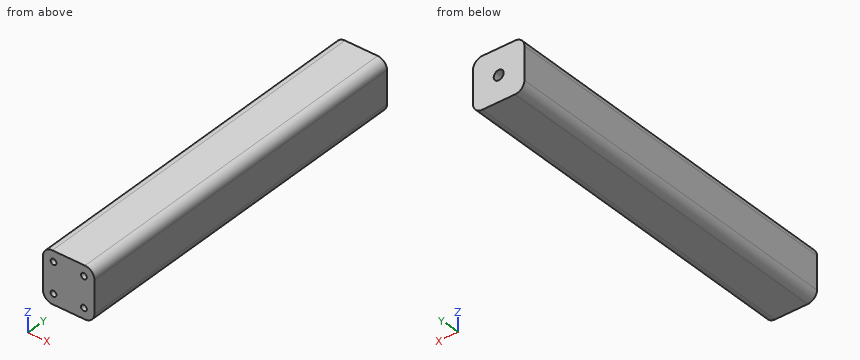
from build123d import *

# Parameters (mm, degrees)
SKETCH_2_W              = 44
SKETCH_2_H              = 44
EXTRUDE_1_DEPTH         = 310
HOLE_WIZARD_M10_1_D     = 8.5
HOLE_WIZARD_M10_1_DEPTH = 25
HOLE_WIZARD_M10_1_TIP   = 2.553657631
HOLE_WIZARD_M6_1_D      = 5
HOLE_WIZARD_M6_1_DEPTH  = 40
HOLE_WIZARD_M6_1_TIP    = 1.502151548
FILLET_1_R              = 8


with BuildPart() as part:
    # 草图2 → 凸台-拉伸1 (new body)
    with BuildSketch(Plane(origin=(0, 0, 0), x_dir=(1, 0, 0), z_dir=(0, 1, 0))):
        with Locations((-0.001355374, -3.30438103)):
            Rectangle(SKETCH_2_W, SKETCH_2_H)
    extrude(amount=EXTRUDE_1_DEPTH)

    # M10 螺纹孔1
    with Locations(Plane(origin=(0, 310, 0), x_dir=(1, 0, 0), z_dir=(0, 1, 0))):
        with Locations((-0.001355374, -3.30438103)):
            Hole(HOLE_WIZARD_M10_1_D / 2, depth=HOLE_WIZARD_M10_1_DEPTH)
            with Locations((0, 0, -(HOLE_WIZARD_M10_1_DEPTH + HOLE_WIZARD_M10_1_TIP / 2))):  # 118° drill point
                Cone(0, HOLE_WIZARD_M10_1_D / 2, HOLE_WIZARD_M10_1_TIP, mode=Mode.SUBTRACT)

    # M6 螺纹孔1
    with Locations(Plane(origin=(-13.001355374, 0, 16.30438103), x_dir=(0, 0, -1), z_dir=(0, -1, 0))):
        with Locations((0, 0), (0, 26), (26, 26), (26, 0)):
            Hole(HOLE_WIZARD_M6_1_D / 2, depth=HOLE_WIZARD_M6_1_DEPTH)
            with Locations((0, 0, -(HOLE_WIZARD_M6_1_DEPTH + HOLE_WIZARD_M6_1_TIP / 2))):  # 118° drill point
                Cone(0, HOLE_WIZARD_M6_1_D / 2, HOLE_WIZARD_M6_1_TIP, mode=Mode.SUBTRACT)

    # 圆角1
    fillet_1_edges = [part.edges().sort_by_distance(p)[0] for p in [
        (-22.001355374, 155, -18.69561897),
        (21.998644626, 155, -18.69561897),
        (21.998644626, 155, 25.30438103),
        (-22.001355374, 155, 25.30438103),
    ]]
    fillet(fillet_1_edges, radius=FILLET_1_R)


solid = part.part
The listing builds one solid part. Answer for the finished solid, in the listing's coordinates (mm). Coordinates: 2 decimals unless noted, no trailing zeros. Write each loop counter-clockwise with the first axis right and the second up, starting at its lowest first coordinate (ties: lowest second). Pieces come first, ordered by that corner, then holes. Notation, with made-up numbers: M 39.25,-17.5 L 86.25,-17.5 A31 ccw 86.25,19.5 Z; hole C -19.75,14.5 d1. An arc over 180 degrees is marked long. Use one line per item in the form item = value.
Item 1: Find the intervals of material crossed by probe 1 along Z at (x, y) = (-12.5, 18); probe 2 along X at (y, z) = (31.5, 16); probe 3 along X at (y, z) = (20, -8.5), in increasing order.
Model answer:
probe_1 = -18.7 to -12.14, -7.25 to 13.86, 18.75 to 25.3
probe_2 = -22 to -15.48, -10.52 to 10.52, 15.48 to 22
probe_3 = -22 to -15.2, -10.81 to 10.8, 15.19 to 22
Item 2: Given P1, Ø4, axis at x = 13, z = -9.7, coming from the -Y side; P2, Ø5, axis at y = 118, z = 20.5, coming from the -X side; P3, Ø3, axis at x = 13, z = 16.3, coming from the -Y side, each flat-ended and moving along its own axis, determine where each tip first touches the part or whether it passes through.
Model answer:
P1 = 40.3
P2 = -21.97
P3 = 40.6
Item 3: Find section B-B, the plane z = 22. Give the vertices of the cut face in (x, y).
Model answer:
outline = M -20.48,0 L 20.48,0 L 20.48,310 L -20.48,310 Z
Item 4: Find section A-A, the plane y = 98.5. Give the vertices of the cut face in (x, z).
Model answer:
outline = M -22,-10.7 A8 ccw -14,-18.7 L 14,-18.7 A8 ccw 22,-10.7 L 22,17.3 A8 ccw 14,25.3 L -14,25.3 A8 ccw -22,17.3 Z
